Design review of the part shown in the three views and the two pictorial views. Dimensions are in mm from the part's minimum x, y and z. A direction names the side the tool comes from. Round coordinates to 2 decimals unless told otherwise and drop trailing zeros. Loops run counter-clockwise (first coordinate to the right, second up) from the corner with the lowest first, then second, coordinate; pieces in that order, holes last. Notation, with made-up numbers: (30, 12.5) -> (78, 12.5) arc R28 cw to (78, 41.5) -> close; hole circle Ø11 at (86.25, 48). An arc over 180 degrees is marked (long way). Use a Markdown table: item, result. Add a question column.
1) Wall thickness on probe 1 along Y at (x, z) = (29, 81); probe 2 along X at (y, z) = (25, 83); probe 3 along Z at (x, y) = (15, 9.5): over which ranges is each line inside the solid? List them lowest first.
2) Consider section C-C on y = 17. Give the boundary of the cut face in (x, z), plus the area to 4 significant figures.
3) Consider section D-D on z = 77. Give the boundary of the cut face in (x, y).
4) Consider section B-B on y = 4.75. Give the boundary of the cut face in (x, z).
5) Consider section A-A on x = 29.25. Give the boundary of the cut face in (y, z).
6) Mouldability with a two-part tool opening along Z and no side actions: class the marked faces 3, 4, 5 and 6 as released by +Z, released by -Z, zero draft, split by the parting line, or undercut.
7) For the marked faces 1 and 2, list the 3-axis set-ups (+Z, -Z, +X, -X, +Y, -Y) from which the entire face can be reached by the end or side of a thin tool; tool diameter is ignored.
8) Insertion check: pin 1 (3 mm diameter, centred on y = 11, z = 66, fed in from -X); pin 2 (3.5 mm diameter, centred on x = 29.25, y = 25.25, fed in from +Z). Each pin has a flat end and moves straight along its axis. Give the tip position at first contact, or say it passes through.
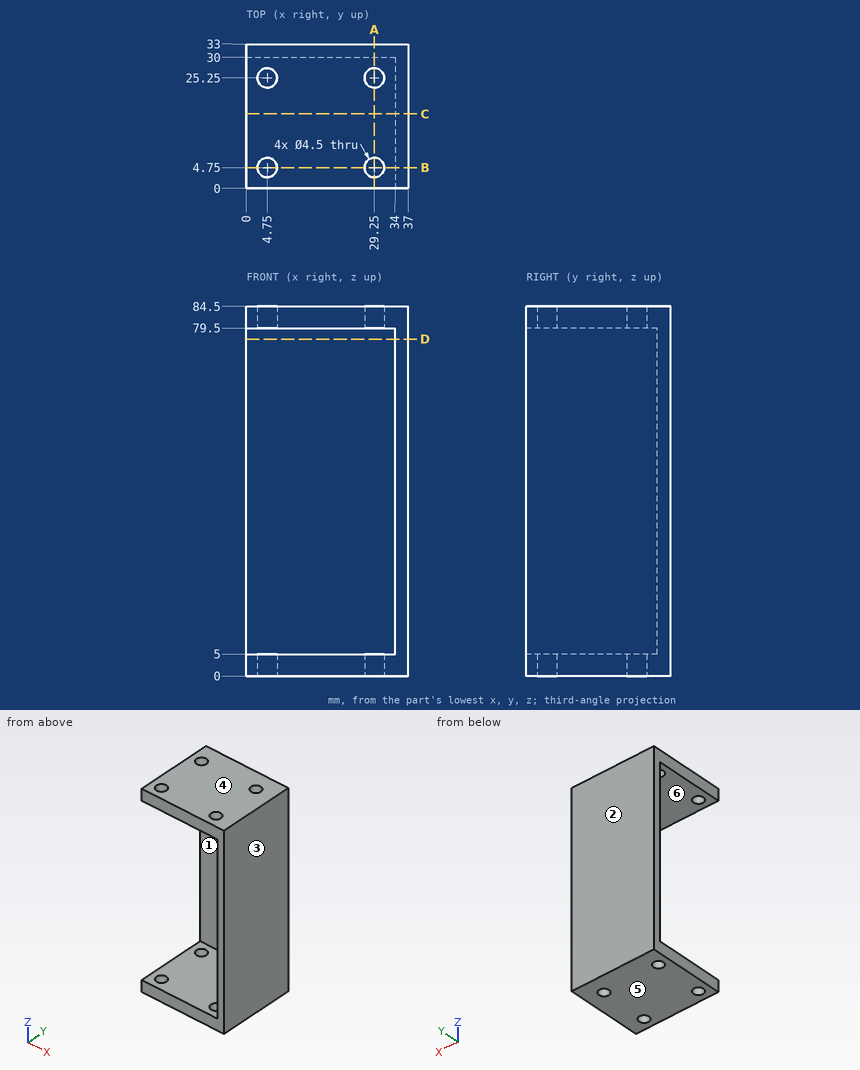
Result set:
| question | item | result |
|---|---|---|
| 1 | probe 1 | 0 to 2.51, 6.99 to 23.01, 27.49 to 33 |
| 1 | probe 2 | 0 to 2.51, 6.99 to 27.01, 31.49 to 37 |
| 1 | probe 3 | 0 to 5, 79.5 to 84.5 |
| 2 | outline | (0, 0) -> (37, 0) -> (37, 84.5) -> (0, 84.5) -> (0, 79.5) -> (34, 79.5) -> (34, 5) -> (0, 5) -> close |
| 2 | area | 593.5 mm2 |
| 3 | outline | (0, 30) -> (34, 30) -> (34, 0) -> (37, 0) -> (37, 33) -> (0, 33) -> close |
| 4 | outline | (0, 0) -> (2.5, 0) -> (2.5, 5) -> (0, 5) -> close; (0, 79.5) -> (2.5, 79.5) -> (2.5, 84.5) -> (0, 84.5) -> close; (7, 0) -> (27, 0) -> (27, 5) -> (7, 5) -> close; (7, 79.5) -> (27, 79.5) -> (27, 84.5) -> (7, 84.5) -> close; (31.5, 0) -> (37, 0) -> (37, 84.5) -> (31.5, 84.5) -> (31.5, 79.5) -> (34, 79.5) -> (34, 5) -> (31.5, 5) -> close |
| 5 | outline | (0, 0) -> (2.5, 0) -> (2.5, 5) -> (0, 5) -> close; (0, 79.5) -> (2.5, 79.5) -> (2.5, 84.5) -> (0, 84.5) -> close; (7, 0) -> (23, 0) -> (23, 5) -> (7, 5) -> close; (7, 79.5) -> (23, 79.5) -> (23, 84.5) -> (7, 84.5) -> close; (27.5, 0) -> (33, 0) -> (33, 84.5) -> (27.5, 84.5) -> (27.5, 79.5) -> (30, 79.5) -> (30, 5) -> (27.5, 5) -> close |
| 6 | face 3 | zero draft |
| 6 | face 4 | released by +Z |
| 6 | face 5 | released by -Z |
| 6 | face 6 | undercut |
| 7 | face 1 | -X, -Y |
| 7 | face 2 | +Z, -Z, +X, -X, +Y |
| 8 | pin 1 | x = 34 |
| 8 | pin 2 | through |
